```python
from build123d import *

# Parameters (mm, degrees)
SKETCH_2_R               = 137.5
SKETCH_2_R_2             = 117.5
EXTRUDE_1_DEPTH          = 10
SKETCH_3_R               = 137.5
EXTRUDE_2_DEPTH          = 20
SKETCH_4_R               = 97.5
CUT_EXTRUDE_1_DEPTH      = 196.480178023
CUT_EXTRUDE_2_DEPTH      = 197.7549237
CUT_EXTRUDE_2_DEPTH_BACK = 197.7549237
SKETCH_6_R               = 5


with BuildPart() as part:
    # 草图2 → 凸台-拉伸1 (new body)
    with BuildSketch(Plane(origin=(0, 0, 0), x_dir=(1, 0, 0), z_dir=(0, 1, 0))):
        with Locations(Location((0, 0, 0), (0, 0, 270))):
            Circle(SKETCH_2_R)
        with Locations(Location((0, 0, 0), (0, 0, 270))):
            Circle(SKETCH_2_R_2, mode=Mode.SUBTRACT)
    extrude(amount=EXTRUDE_1_DEPTH)

    # 草图3 → 凸台-拉伸2 (add)
    with BuildSketch(Plane(origin=(0, 10, 0), x_dir=(1, 0, 0), z_dir=(0, 1, 0))):
        with Locations(Location((0, 0, 0), (0, 0, 270))):
            Circle(SKETCH_3_R)
    extrude(amount=EXTRUDE_2_DEPTH)

    # 草图4 → 切除-拉伸1 (cut, through all)
    with BuildSketch(Plane.XZ.offset(-10)):
        with Locations(Location((0, 0, 0), (0, 0, 270))):
            Circle(SKETCH_4_R)
    extrude(amount=-CUT_EXTRUDE_1_DEPTH, mode=Mode.SUBTRACT)

    # 草图6 → 切除-拉伸2 (cut, two sides: drawn at the far end of the back side and taken through both)
    with BuildSketch(Plane(origin=(0, 30, 0), x_dir=(1, 0, 0), z_dir=(0, 1, 0)).offset(-CUT_EXTRUDE_2_DEPTH_BACK)):
        with Locations(Location((80.922446863, 66.907081792, 0), (0, 0, 270))):
            Circle(SKETCH_6_R)
        with Locations(Location((66.907081793, -80.922446862, 0), (0, 0, 270))):
            Circle(SKETCH_6_R)
        with Locations(Location((-80.922446861, -66.907081792, 0), (0, 0, 270))):
            Circle(SKETCH_6_R)
        with Locations(Location((-66.907081791, 80.922446862, 0), (0, 0, 270))):
            Circle(SKETCH_6_R)
    extrude(amount=CUT_EXTRUDE_2_DEPTH + CUT_EXTRUDE_2_DEPTH_BACK, mode=Mode.SUBTRACT)


solid = part.part
```
Check sheet for the modelled part. Datum: model origin and axes. Units: mm. A direction names the side the tool comes from. Give positions to 0.01 mm unless a question says otherwise; leave off trailing zeros. Write each loop counter-clockwise with the first axis right and the second up, starting at its lowest first coordinate (ties: lowest second). Pieces come first, ordered by that corner, then holes.
Item 1: Cross-section at A-A (x = 0). Enter the section's corners in (y, z).
Item 2: Cross-section at D-D (y = 22). Enter the section's corners in (x, z), and give its area (3 significant figures).
Item 3: Gauge pin test, flat ends, axial feed: pin 1 (11.5 mm diameter, centred on x = 66.91, z = 80.92, fed in from +Y); pin 2 (11.5 mm diameter, centred on x = 80.92, z = -66.91, fed in from -Y); pin 3 (8 mm diameter, centred on x = -66.91, z = -80.92, fed in from -Y); pin 4 (4 mm diameter, centred on y = 22.5, z = 78, fed in from -X). Record the tip position at first contact, or that the pin passes through.
Item 4: Scan lines: L1, parallel to Z at x = 71.5, y = 19.75; L2, parallel to X at y = 16, z = 71; L3, parallel to X at y = 18.75, z = -15. Record each from-to range of solid material in increasing order.
Item 5: Cross-section at B-B (z = -58.5). Enter the section's corners in (x, y).
Item 6: Access from +Z, -Z, +X, -X, +Y, -Y to the whole of each face (thin tool, end or side, straight path). Record for faces 1 (the face through (88, 10, -44)), 2 (the face through (76.04, 19.86, -67.99)).
Item 7: Draft check along X on faces 3 (the face through (-85.8, 19.9, 65.8)), 4 (the face through (62, 0, 101)), 5 (the face through (41.3, 14.79, 131.15)). Enter one of: released by +X, released by -X, zero draft, split by the parting line, or undercut.
Item 8: Cross-section at C-C (y = 6.5). Enter the section's corners in (x, z).
Report:
1. outline: (0, -137.5) - (30, -137.5) - (30, -97.5) - (10, -97.5) - (10, -117.5) - (0, -117.5) - close; (0, 117.5) - (10, 117.5) - (10, 97.5) - (30, 97.5) - (30, 137.5) - (0, 137.5) - close
2. outline: circle Ø275 at (0, 0); hole circle Ø195 at (0, 0); hole circle Ø10 at (-80.92, 66.91); hole circle Ø10 at (-66.91, -80.92); hole circle Ø10 at (66.91, 80.92); hole circle Ø10 at (80.92, -66.91)
2. area: 29,200 mm2
3. pin 1: stops at y = 30
3. pin 2: stops at y = 10
3. pin 3: passes through
3. pin 4: stops at x = -114.59
4. L1: z = -117.45 to -66.29, 66.29 to 78.95, 82.9 to 117.45
4. L2: x = -117.75 to -83.79, -78.05 to -66.82, 66.82 to 117.75
4. L3: x = -136.68 to -96.34, 96.34 to 136.68
5. outline: (-124.43, 0) - (-101.9, 0) - (-101.9, 10) - (-78, 10) - (-78, 30) - (-124.43, 30) - close; (78, 10) - (101.9, 10) - (101.9, 0) - (124.43, 0) - (124.43, 30) - (78, 30) - close
6. face 1: -Y
6. face 2: +Y, -Y
7. face 3: undercut
7. face 4: zero draft
7. face 5: split by the parting line
8. outline: circle Ø275 at (0, 0); hole circle Ø235 at (0, 0)
